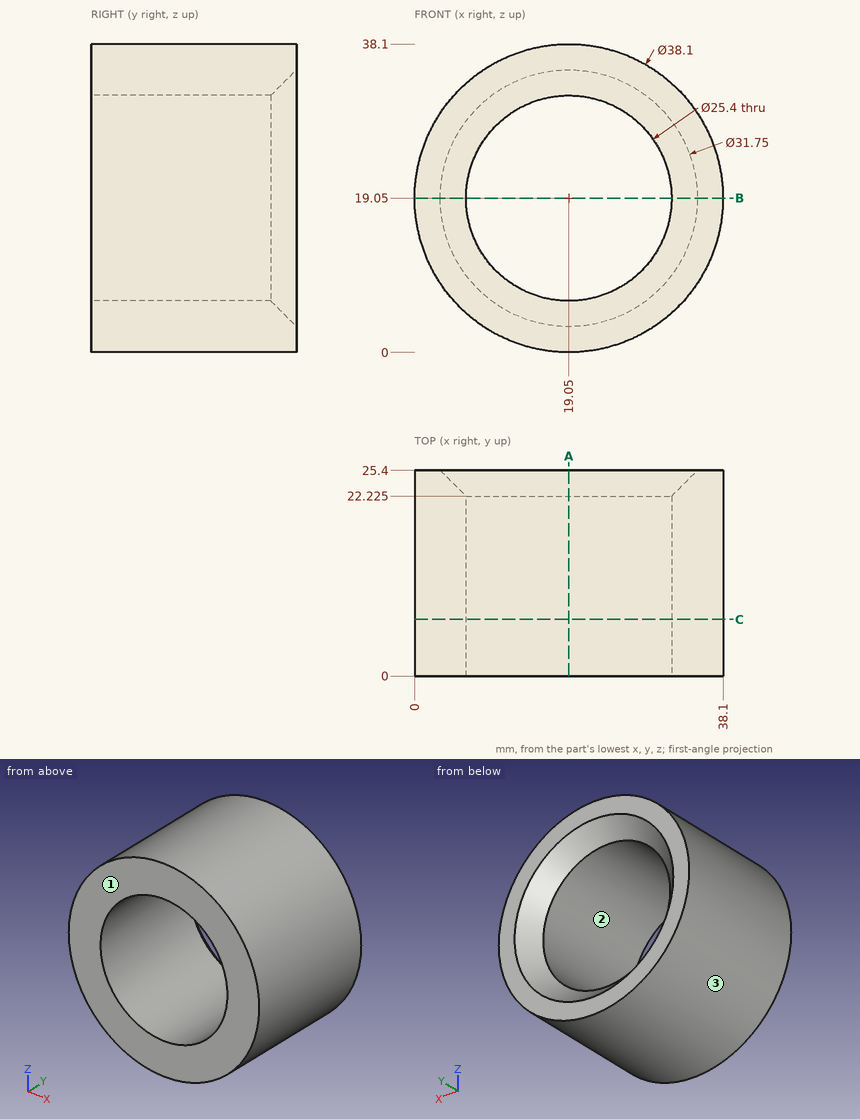
Drawing for the job (mm, zero at the part's lowest x, y, z). Give positions to 0.01 mm unless a question says otherwise; leave off trailing zeros. Loops run counter-clockwise (first coordinate to the right, second up) from the corner with the lowest first, then second, coordinate; pieces in that order, holes last. Notation, with made-up numbers: (-34, 74.25) - (11, 74.25) arc R25 ccw to (11, 107.25) - close; hole circle Ø4 at (16, -38.75). An arc over 180 degrees is marked (long way). Write item = value, one per line. Start each with the question number.
1) Band-saw the part on A-A on x = 19.05. Give the cut face in (y, z) (3 decimals).
2) Drop flat-ended pins along their axis: pin 1 Ø8 at (y, z) = (15, 33) entering from -X (3 decimals); pin 2 Ø2 at (x, y) = (15, 14) entering from +Z; pin 3 Ø12 at (y, z) = (6, 32.5) entering from +X; pin 4 Ø20.5 at (x, z) = (19.05, 19.05) entering from +Y. Give the stop position or say it passes through.
3) Probe probe 1 along Z at (x, y) = (19.05, 12.25); probe 2 along X at (y, z) = (14, 24); probe 3 along X at (y, z) = (23.25, 25.5) (3 decimals). List the from-to ranges inside material, lowest first. Write a range as from..to.
4) Pull direction X, two halves, no side cores. Call the marked faces 1, 2 and 3: +X half, -X half, draft (parallel to the pull), parting line (faces both ways), or undercut.
5) Band-saw the part on C-C on y = 7. Give the cut face in (x, z).
6) Band-saw the part on B-B on z = 19.05. Give the cut face in (x, y) (3 decimals), plus the area to 4 significant figures.
Final values:
q1.outline = (0, 0) - (25.4, 0) - (25.4, 3.175) - (22.225, 6.35) - (0, 6.35) - close; (0, 31.75) - (22.225, 31.75) - (25.4, 34.925) - (25.4, 38.1) - (0, 38.1) - close
q2.pin_1 = 2.805
q2.pin_2 = 37.85
q2.pin_3 = 36.58
q2.pin_4 = through
q3.probe_1 = 0..6.35, 31.75..38.1
q3.probe_2 = 0.65..7.35, 30.75..37.45
q3.probe_3 = 1.125..6.935, 31.165..36.975
q4.face_1 = draft
q4.face_2 = undercut
q4.face_3 = parting line
q5.outline = circle Ø38.1 at (19.05, 19.05); hole circle Ø25.4 at (19.05, 19.05)
q6.outline = (0, 0) - (6.35, 0) - (6.35, 22.225) - (3.175, 25.4) - (0, 25.4) - close; (31.75, 0) - (38.1, 0) - (38.1, 25.4) - (34.925, 25.4) - (31.75, 22.225) - close
q6.area = 312.5 mm²
